Source: CAD feature listing. Evaluate the final solid. Frame: model axes, mm. A direction names the side the tool comes from. Give positions to 0.01 mm unless a question says otherwise; leave off trailing zeros. Loops run counter-clockwise (first coordinate to the right, second up) from the corner with the lowest first, then second, coordinate; pieces in that order, holes last.
from build123d import *

# Parameters (mm, degrees)
SKETCH1_W          = 300
SKETCH1_H          = 250
BASE_DEPTH         = 14
SKETCH3_W          = 240
SKETCH3_H          = 230
CUT_EXTRUDE1_DEPTH = 10
FILLET1_R          = 5
FILLET2_R          = 5
SKETCH4_W          = 240
SKETCH4_H          = 80
DIN_BASE_DEPTH     = 10
SKETCH5_W          = 10
SKETCH5_H          = 70
DIN_STAND_DEPTH    = 50


with BuildPart() as part:
    # Sketch1 → Base (new body)
    with BuildSketch(Plane(origin=(0, 0, 0), x_dir=(1, 0, 0), z_dir=(0, 1, 0))):
        Rectangle(SKETCH1_W, SKETCH1_H)
    extrude(amount=BASE_DEPTH)

    # Sketch3 → Cut-Extrude1 (cut)
    with BuildSketch(Plane(origin=(0, 14, 0), x_dir=(1, 0, 0), z_dir=(0, 1, 0))):
        Rectangle(SKETCH3_W, SKETCH3_H)
    extrude(amount=-CUT_EXTRUDE1_DEPTH, mode=Mode.SUBTRACT)

    # Fillet1
    fillet1_edges = [part.edges().sort_by_distance(p)[0] for p in [
        (0, 0, 125),
        (-150, 0, 0),
        (0, 0, -125),
        (150, 0, 0),
    ]]
    fillet(fillet1_edges, radius=FILLET1_R)

    # Fillet2
    # the kernel refuses this fillet: 5 mm, written as the material it takes off along each edge
    with BuildSketch(Plane(origin=(145, 5, 120), x_dir=(1, 0, 0), z_dir=(0, 0, 1))) as fillet2_piece_1_section:
        Polygon((0, 0), (FILLET2_R, 0), (FILLET2_R, -FILLET2_R), (0, -FILLET2_R), align=None)
    fillet2_piece_1 = extrude(amount=FILLET2_R, mode=Mode.PRIVATE)
    fillet2_piece_1 = fillet2_piece_1 - Plane(origin=(145, 5, 120), x_dir=(-0.7071067811865475, 0.7071067811865475, 0), z_dir=(0, 0, 1)) * Sphere(FILLET2_R, mode=Mode.PRIVATE)
    add(fillet2_piece_1, mode=Mode.SUBTRACT)
    with BuildSketch(Plane(origin=(-145, 5, 120), x_dir=(-1, 0, 0), z_dir=(0, 0, 1))) as fillet2_piece_2_section:
        Polygon((0, 0), (FILLET2_R, 0), (FILLET2_R, FILLET2_R), (0, FILLET2_R), align=None)
    fillet2_piece_2 = extrude(amount=FILLET2_R, mode=Mode.PRIVATE)
    fillet2_piece_2 = fillet2_piece_2 - Plane(origin=(-145, 5, 120), x_dir=(0.7071067811865475, 0.7071067811865475, 0), z_dir=(0, 0, 1)) * Sphere(FILLET2_R, mode=Mode.PRIVATE)
    add(fillet2_piece_2, mode=Mode.SUBTRACT)
    with BuildSketch(Plane(origin=(145, 5, -120), x_dir=(0, 0, -1), z_dir=(1, 0, 0))) as fillet2_piece_3_section:
        Polygon((0, 0), (FILLET2_R, 0), (FILLET2_R, -FILLET2_R), (0, -FILLET2_R), align=None)
    fillet2_piece_3 = extrude(amount=FILLET2_R, mode=Mode.PRIVATE)
    fillet2_piece_3 = fillet2_piece_3 - Plane(origin=(145, 5, -120), x_dir=(0, 0.7071067811865475, 0.7071067811865475), z_dir=(1, 0, 0)) * Sphere(FILLET2_R, mode=Mode.PRIVATE)
    add(fillet2_piece_3, mode=Mode.SUBTRACT)
    with BuildSketch(Plane(origin=(-145, 5, -120), x_dir=(0, 0, -1), z_dir=(-1, 0, 0))) as fillet2_piece_4_section:
        Polygon((0, 0), (FILLET2_R, 0), (FILLET2_R, FILLET2_R), (0, FILLET2_R), align=None)
    fillet2_piece_4 = extrude(amount=FILLET2_R, mode=Mode.PRIVATE)
    fillet2_piece_4 = fillet2_piece_4 - Plane(origin=(-145, 5, -120), x_dir=(0, 0.7071067811865475, 0.7071067811865475), z_dir=(-1, 0, 0)) * Sphere(FILLET2_R, mode=Mode.PRIVATE)
    add(fillet2_piece_4, mode=Mode.SUBTRACT)
    with BuildSketch(Plane(origin=(150, 5, 125), x_dir=(-1, 0, 0), z_dir=(0, 1, 0)), Plane(origin=(150, 5, -125), x_dir=(0, 0, 1), z_dir=(0, 1, 0))) as fillet2_piece_5:
        with BuildLine():
            CenterArc((FILLET2_R, -FILLET2_R), FILLET2_R, 90, 90)
            Line((0, -FILLET2_R), (0, 0))
            Line((0, 0), (FILLET2_R, 0))
        make_face()
    extrude(amount=21.5, mode=Mode.SUBTRACT)
    with BuildSketch(Plane(origin=(-150, 5, 125), x_dir=(1, 0, 0), z_dir=(0, 1, 0)), Plane(origin=(-150, 5, -125), x_dir=(0, 0, 1), z_dir=(0, 1, 0))) as fillet2_piece_6:
        with BuildLine():
            CenterArc((FILLET2_R, FILLET2_R), FILLET2_R, 180, 90)
            Line((0, FILLET2_R), (0, 0))
            Line((0, 0), (FILLET2_R, 0))
        make_face()
    extrude(amount=21.5, mode=Mode.SUBTRACT)

    # Sketch4 → DIN Base (add)
    with BuildSketch(Plane(origin=(0, 4, 0), x_dir=(1, 0, 0), z_dir=(0, 1, 0))):
        with Locations((0, 20)):
            Rectangle(SKETCH4_W, SKETCH4_H)
    extrude(amount=DIN_BASE_DEPTH)

    # Sketch5 → DIN Stand (add)
    with BuildSketch(Plane(origin=(0, 14, 0), x_dir=(1, 0, 0), z_dir=(0, 1, 0))):
        with Locations((135, 20)):
            Rectangle(SKETCH5_W, SKETCH5_H)
        with Locations((-10, 20)):
            Rectangle(SKETCH5_W, SKETCH5_H)
    extrude(amount=DIN_STAND_DEPTH)


solid = part.part
1) Contact query for flat-ended pins moving along their axis: P1, Ø11, axis at x = 136.5, y = 39, coming from the -Z side; P2, Ø8, axis at y = 45.5, z = -25.5, coming from the +X side; P3, Ø10, axis at y = 22.5, z = 59, coming from the -X side; P4, Ø8, axis at x = 136.5, y = 47, coming from the +Z side. Output: stop coordinate, or through.
Checks:
P1: stops at z = -55
P2: stops at x = 140
P3: passes through
P4: stops at z = 15
2) Cut plane D-D (y = 9). Return loops of the section in (x, z), and give its area (3 significant figures).
Checks:
outline: (-150, -120) arc R5 ccw to (-145, -125) - (145, -125) arc R5 ccw to (150, -120) - (150, 120) arc R5 ccw to (145, 125) - (-145, 125) arc R5 ccw to (-150, 120) - close; hole (-120, -115) - (120, -115) - (120, -60) - (-120, -60) - close; hole (-120, 20) - (120, 20) - (120, 115) - (-120, 115) - close
area: 39,000 mm2
3) Reachability of faces 1 (the flat face through (-10, 39, 15)), 2 (the flat face through (-10, 39, -55)), 3 (the flat face through (-2, 9, 125)), 4 (the flat face through (120, 9, 68)) from +Z, -Z, +X, -X, +Y, -Y: full face, straight path, thin tool, end or side. Return the list, or none.
Checks:
face 1: +Z, +X, -X, +Y
face 2: -Z, +X, -X, +Y
face 3: +Z, +X, -X, +Y, -Y
face 4: +Y
4) Cut plane A-A (y = 44). Return loops of the section in (x, z).
Checks:
outline: (-15, -55) - (-5, -55) - (-5, 15) - (-15, 15) - close; (130, -55) - (140, -55) - (140, 15) - (130, 15) - close
5) Ray query, probe 1 along Z at (x, y) = (-29, 5); probe 2 along X at (y, z) = (7, -78); probe 3 along X at (y, z) = (21.5, 5). Return the intervals inside material, ascending.
Checks:
probe 1: z = -125 to -115, -60 to 20, 115 to 125
probe 2: x = -150 to -120, 120 to 150
probe 3: x = -15 to -5, 130 to 140
6) Cut plane B-B (z = -9). Return loops of the section in (x, y).
Checks:
outline: (-150, 5) arc R5 ccw to (-145, 0) - (145, 0) arc R5 ccw to (150, 5) - (150, 14) - (140, 14) - (140, 64) - (130, 64) - (130, 14) - (-5, 14) - (-5, 64) - (-15, 64) - (-15, 14) - (-150, 14) - close
7) Cut plane C-C (x = -49.5). Return loops of the section in (y, z), and give its area (3 significant figures).
Checks:
outline: (0, -120) arc R5 ccw to (5, -125) - (14, -125) - (14, -115) - (4, -115) - (4, -60) - (14, -60) - (14, 20) - (4, 20) - (4, 115) - (14, 115) - (14, 125) - (5, 125) arc R5 ccw to (0, 120) - close
area: 1,990 mm2
8) Pull-direction query (X, two-part tool) for faces 5 (the flat face through (130, 39, -20)), 6 (the flat face through (-10, 64, -20)), 7 (the flat face through (140, 39, -20)), 8 (the flat face through (-2, 9, -115)); classes: released by +X, released by -X, zero draft, split by the parting line, or undercut.
Checks:
face 5: undercut
face 6: zero draft
face 7: released by +X
face 8: undercut
